Check sheet for the modelled part. Datum: model origin and axes. Units: mm. A direction names the side the tool comes from. Coordinates: 2 decimals unless noted, no trailing zeros. Loops run counter-clockwise (first coordinate to the right, second up) from the corner with the lowest first, then second, coordinate; pieces in that order, holes last. Notation, with made-up numbers: (11.25, 69) -> (42.25, 69) arc R27 ccw to (42.25, 86) -> close; hole circle Ø11 at (34, 18.25). An arc over 180 degrees is marked (long way). Use CSV: the item, a comma, the result in double quotes. Start each with the question number.
1. Sectioned sample at B-B, the plane x = 0. Record the cut outline in (y, z), and give its area (3 significant figures).
2. Thickness scan on L1, parallel to X at y = 0, z = 2.7; L2, parallel to X at y = 12, z = 1; L3, parallel to Y at x = -4, z = 1. Record the ranges inside material, lowest first.
3. Set-up check for faces 1 (the face through (-16, 1.119, 3)), 2 (the face through (16.45, 0, 3)), 3 (the face through (16, -1.119, 3)): record each of +Z, -Z, +X, -X, +Y, -Y from which the full face is reachable in a straight line by a thin tool's end or side.
4. Gauge pin test, flat ends, axial feed: pin 1 (1 mm diameter, centred on y = -6.5, z = 1, fed in from +X); pin 2 (2 mm diameter, centred on x = -7.5, z = 1.5, fed in from -Y); pin 3 (2 mm diameter, centred on x = -11, z = 2, fed in from -Y). Record the tip position at first contact, or that the pin passes through.
5. Release check for a two-part mould opening along X. For faces 4 (the face through (-16.45, 0, 3)), 5 (the face through (15.243, -0.449, 1.083)), 6 (the face through (-6.3, 14.1, 2)) record: pulls with the +X half, pulls with the -X half, needs draft (parallel to the pull), parting line crosses it, or undercut.
6. Sectioned sample at C-C, the plane y = 0. Record the cut outline in (x, z).
7. Sectioned sample at A-A, the plane z = 3. Record the cut outline in (x, y), and give its area (3 significant figures).
```python
from build123d import *

# Parameters (mm, degrees)
F0_R     = 25
F1_DEPTH = 2
F3_DEPTH = 4


# Not quite as in the source:
# - a fillet or chamfer that OpenCascade refuses, or shapes differently, is made with other operations: its cross-section is extruded or revolved along the edge and cut away or added


with BuildPart() as f1:
    # F0 (on Top) → F1 (new body)
    with BuildSketch(Plane.XY):
        Circle(F0_R)
        with BuildLine():
            ThreePointArc((-15.2089073237, 1.1187662932), (0, 15.25), (15.2089073237, 1.1187662932))
            Line((15.2089073237, 1.1187662932), (16.45, 1.1187662932))
            Line((16.45, 1.1187662932), (16.45, -1.1187662932))
            Line((16.45, -1.1187662932), (15.2089073237, -1.1187662932))
            ThreePointArc((15.2089073237, -1.1187662932), (0, -15.25), (-15.2089073237, -1.1187662932))
            Line((-15.2089073237, -1.1187662932), (-16.45, -1.1187662932))
            Line((-16.45, -1.1187662932), (-16.45, 1.1187662932))
            Line((-16.45, 1.1187662932), (-15.2089073237, 1.1187662932))
        make_face(mode=Mode.SUBTRACT)
        with BuildLine():
            ThreePointArc((15.2089073237, 1.1187662932), (15.2397233683, 0.5597603565), (15.25, 0))
            ThreePointArc((15.25, 0), (15.2397233683, -0.5597603565), (15.2089073237, -1.1187662932))
            Line((15.2089073237, -1.1187662932), (16.45, -1.1187662932))
            Line((16.45, -1.1187662932), (16.45, 1.1187662932))
            Line((16.45, 1.1187662932), (15.2089073237, 1.1187662932))
        make_face()
        with BuildLine():
            ThreePointArc((-15.2089073237, -1.1187662932), (-15.25, 0), (-15.2089073237, 1.1187662932))
            Line((-15.2089073237, 1.1187662932), (-16.45, 1.1187662932))
            Line((-16.45, 1.1187662932), (-16.45, -1.1187662932))
            Line((-16.45, -1.1187662932), (-15.2089073237, -1.1187662932))
        make_face()
    extrude(amount=F1_DEPTH)

    # F2: fillet of radius 5 on 1 edges, made by hand

    # F2_s1 → F2_t2 (revolve, cut)
    with BuildSketch(Plane.XZ):
        with BuildLine():
            ThreePointArc((25, 0), (23.2360679775, 1.472135955), (21, 2))
            Line((21, 2), (25, 2))
            Line((25, 2), (25, 0))
        make_face()
    revolve(axis=Axis((0, 0, 2), (0, 0, 1)), mode=Mode.SUBTRACT)

    # F0 (on Top) → F3 (join)
    with BuildSketch(Plane.XY):
        with BuildLine():
            ThreePointArc((15.2089073237, 1.1187662932), (15.2397233683, 0.5597603565), (15.25, 0))
            ThreePointArc((15.25, 0), (15.2397233683, -0.5597603565), (15.2089073237, -1.1187662932))
            Line((15.2089073237, -1.1187662932), (16.45, -1.1187662932))
            Line((16.45, -1.1187662932), (16.45, 1.1187662932))
            Line((16.45, 1.1187662932), (15.2089073237, 1.1187662932))
        make_face()
        with BuildLine():
            ThreePointArc((-15.2089073237, -1.1187662932), (-15.25, 0), (-15.2089073237, 1.1187662932))
            Line((-15.2089073237, 1.1187662932), (-16.45, 1.1187662932))
            Line((-16.45, 1.1187662932), (-16.45, -1.1187662932))
            Line((-16.45, -1.1187662932), (-15.2089073237, -1.1187662932))
        make_face()
    extrude(amount=F3_DEPTH)


solid = f1.part
```
Completed:
1,outline,"(-25, 0) -> (-15.25, 0) -> (-15.25, 2) -> (-21, 2) arc R5 ccw to start; (15.25, 0) -> (25, 0) arc R5 ccw to (21, 2) -> (15.25, 2) -> close"
1,area,"34.2 mm²"
2,L1,"-16.45 to -15.25, 15.25 to 16.45"
2,L2,"-20.78 to -9.41, 9.41 to 20.78"
2,L3,"-23.66 to -14.72, 14.72 to 23.66"
3,face 1,"+Z, +X, -X, +Y"
3,face 2,"+Z, +X, +Y, -Y"
3,face 3,"+Z, +X, -X, -Y"
4,pin 1,"x = 23.71"
4,pin 2,"y = -23.44"
4,pin 3,"y = -21.41"
5,face 4,"pulls with the -X half"
5,face 5,"undercut"
5,face 6,"needs draft"
6,outline,"(-25, 0) -> (-15.25, 0) -> (-15.25, 4) -> (-16.45, 4) -> (-16.45, 2) -> (-21, 2) arc R5 ccw to start; (15.25, 0) -> (25, 0) arc R5 ccw to (21, 2) -> (16.45, 2) -> (16.45, 4) -> (15.25, 4) -> close"
7,outline,"(-16.45, -1.12) -> (-15.21, -1.12) arc R15.25 cw to (-15.21, 1.12) -> (-16.45, 1.12) -> close; (15.21, -1.12) -> (16.45, -1.12) -> (16.45, 1.12) -> (15.21, 1.12) arc R15.25 cw to start"
7,area,"5.43 mm²"
